Part model, mm, in its own coordinate system. A direction names the side the tool comes from. Round coordinates to 2 decimals unless told otherwise and drop trailing zeros. Order: outer loops, then holes, each group sorted by start corner. A loop starts at its lowest first (then second) coordinate and runs counter-clockwise, first axis right, second up. Notation, with made-up numbers: (64.5, 14) - (111.5, 14) arc R21 ccw to (111.5, 36) - close; hole circle Ø8 at (16.5, 25.25). An arc over 180 degrees is marked (long way). Return JSON: item names as keys, results as strings. Group by question number.
Item 1: Tool access for faces 1 (the face through (-32.795, -70.53, 4.698)), 2 (the face through (30.354, -69.132, 4.698)), 3 (the face through (41.99, -80.98, 0.49)): list every direction of +Z, -Z, +X, -X, +Y, -Y with a clear straight run to the whole face (end or side of a thin tool).
Item 2: Saw through at C-C on z = 2.5. State how many separate pieces and enclosed holes the cut face has, and give its area (3 significant figures).
Item 3: Probe probe 1 along X at (y, z) = (12, 4.25); probe 2 along Z at (x, y) = (38.5, -73.5); probe 3 along X at (y, z) = (3, 1.75). List the from-to ranges inside material, lowest first.
Item 4: Saw through at B-B on y = 26.5. List the corners of the cut face in (x, z), and give its area (3 significant figures).
Item 5: Drop flat-ended pins along their axis: pin 1 (2 mm diameter, centred on y = -13, z = 3, fed in from +X); pin 2 (4 mm diameter, centred on y = -7, z = 3.5, fed in from -X); pin 3 (3 mm diameter, centred on x = 13.5, z = 3.5, fed in from -Y). Give the stop position or say it passes through.
Item 6: Two-plate mould, pull along Y, no slides. Class faces 4 (the face through (-32.506, -44, 5)), 5 (the face through (-43, 49.31, 0.49)), 6 (the face through (-34.506, -15, 5)): released by +Y, released by -Y, zero draft, split by the parting line, or undercut.
```python
from build123d import *

# Parameters (mm, degrees)
F0_W     = 64
F0_H     = 16.5
F1_DEPTH = 1
F2_DEPTH = 8.5
F0_H_2   = 2
F3_DEPTH = 8.5


with BuildPart() as f1:
    # F0 (on Top) → F1 (new body)
    with BuildSketch(Plane.XY):
        with BuildLine():
            Line((34.994369, 52.165454), (-36.005631, 52.165454))
            ThreePointArc((-36.005631, 52.165454), (-43.076699, 49.236522), (-46.005631, 42.165454))
            Line((-46.005631, 42.165454), (-46.005631, -73.834546))
            ThreePointArc((-46.005631, -73.834546), (-43.076699, -80.905614), (-36.005631, -83.834546))
            Line((-36.005631, -83.834546), (34.994369, -83.834546))
            ThreePointArc((34.994369, -83.834546), (42.065437, -80.905614), (44.994369, -73.834546))
            Line((44.994369, -73.834546), (44.994369, 42.165454))
            ThreePointArc((44.994369, 42.165454), (42.065437, 49.236522), (34.994369, 52.165454))
        make_face()
        with BuildLine():
            ThreePointArc((-38.505631, 34.665454), (-35.576699, 41.736522), (-28.505631, 44.665454))
            Line((-28.505631, 44.665454), (27.494369, 44.665454))
            ThreePointArc((27.494369, 44.665454), (34.565437, 41.736522), (37.494369, 34.665454))
            Line((37.494369, 34.665454), (37.494369, -66.334546))
            ThreePointArc((37.494369, -66.334546), (34.565437, -73.405614), (27.494369, -76.334546))
            Line((27.494369, -76.334546), (-28.505631, -76.334546))
            ThreePointArc((-28.505631, -76.334546), (-35.576699, -73.405614), (-38.505631, -66.334546))
            Line((-38.505631, -66.334546), (-38.505631, 34.665454))
        make_face(mode=Mode.SUBTRACT)
        with BuildLine():
            Line((27.494369, 44.665454), (-28.505631, 44.665454))
            ThreePointArc((-28.505631, 44.665454), (-35.576699, 41.736522), (-38.505631, 34.665454))
            Line((-38.505631, 34.665454), (-38.505631, -66.334546))
            ThreePointArc((-38.505631, -66.334546), (-35.576699, -73.405614), (-28.505631, -76.334546))
            Line((-28.505631, -76.334546), (27.494369, -76.334546))
            ThreePointArc((27.494369, -76.334546), (34.565437, -73.405614), (37.494369, -66.334546))
            Line((37.494369, -66.334546), (37.494369, 34.665454))
            ThreePointArc((37.494369, 34.665454), (34.565437, 41.736522), (27.494369, 44.665454))
        make_face()
        with BuildLine():
            ThreePointArc((-36.505631, 34.665454), (-34.162485, 40.322309), (-28.505631, 42.665454))
            Line((-28.505631, 42.665454), (27.494369, 42.665454))
            ThreePointArc((27.494369, 42.665454), (33.151223, 40.322309), (35.494369, 34.665454))
            Line((35.494369, 34.665454), (35.494369, -66.334546))
            ThreePointArc((35.494369, -66.334546), (33.151223, -71.9914), (27.494369, -74.334546))
            Line((27.494369, -74.334546), (-28.505631, -74.334546))
            ThreePointArc((-28.505631, -74.334546), (-34.162485, -71.9914), (-36.505631, -66.334546))
            Line((-36.505631, -66.334546), (-36.505631, 34.665454))
        make_face(mode=Mode.SUBTRACT)
        with BuildLine():
            Line((27.494369, 42.665454), (-28.505631, 42.665454))
            ThreePointArc((-28.505631, 42.665454), (-34.162485, 40.322309), (-36.505631, 34.665454))
            Line((-36.505631, 34.665454), (-36.505631, -66.334546))
            ThreePointArc((-36.505631, -66.334546), (-34.162485, -71.9914), (-28.505631, -74.334546))
            Line((-28.505631, -74.334546), (27.494369, -74.334546))
            ThreePointArc((27.494369, -74.334546), (33.151223, -71.9914), (35.494369, -66.334546))
            Line((35.494369, -66.334546), (35.494369, 34.665454))
            ThreePointArc((35.494369, 34.665454), (33.151223, 40.322309), (27.494369, 42.665454))
        make_face()
        with BuildLine():
            ThreePointArc((-34.505631, 34.665454), (-32.748272, 38.908095), (-28.505631, 40.665454))
            Line((-28.505631, 40.665454), (27.494369, 40.665454))
            ThreePointArc((27.494369, 40.665454), (31.73701, 38.908095), (33.494369, 34.665454))
            Line((33.494369, 34.665454), (33.494369, -66.334546))
            ThreePointArc((33.494369, -66.334546), (31.73701, -70.577186), (27.494369, -72.334546))
            Line((27.494369, -72.334546), (-28.505631, -72.334546))
            ThreePointArc((-28.505631, -72.334546), (-32.748272, -70.577186), (-34.505631, -66.334546))
            Line((-34.505631, -66.334546), (-34.505631, 34.665454))
        make_face(mode=Mode.SUBTRACT)
        with BuildLine():
            Line((27.494369, 40.665454), (-28.505631, 40.665454))
            ThreePointArc((-28.505631, 40.665454), (-32.748272, 38.908095), (-34.505631, 34.665454))
            Line((-34.505631, 34.665454), (-34.505631, -66.334546))
            ThreePointArc((-34.505631, -66.334546), (-32.748272, -70.577186), (-28.505631, -72.334546))
            Line((-28.505631, -72.334546), (27.494369, -72.334546))
            ThreePointArc((27.494369, -72.334546), (31.73701, -70.577186), (33.494369, -66.334546))
            Line((33.494369, -66.334546), (33.494369, 34.665454))
            ThreePointArc((33.494369, 34.665454), (31.73701, 38.908095), (27.494369, 40.665454))
        make_face()
        with BuildLine():
            ThreePointArc((-32.505631, 34.665454), (-31.334058, 37.493881), (-28.505631, 38.665454))
            Line((-28.505631, 38.665454), (27.494369, 38.665454))
            ThreePointArc((27.494369, 38.665454), (30.322796, 37.493881), (31.494369, 34.665454))
            Line((31.494369, 34.665454), (31.494369, 22.165454))
            Line((31.494369, 22.165454), (31.494369, 20.165454))
            Line((31.494369, 20.165454), (31.494369, 3.665454))
            Line((31.494369, 3.665454), (31.494369, 1.665454))
            Line((31.494369, 1.665454), (31.494369, -14.834546))
            Line((31.494369, -14.834546), (31.494369, -16.834546))
            Line((31.494369, -16.834546), (31.494369, -33.334546))
            Line((31.494369, -33.334546), (31.494369, -35.334546))
            Line((31.494369, -35.334546), (31.494369, -51.834546))
            Line((31.494369, -51.834546), (31.494369, -53.834546))
            Line((31.494369, -53.834546), (31.494369, -66.334546))
            ThreePointArc((31.494369, -66.334546), (30.322796, -69.162973), (27.494369, -70.334546))
            Line((27.494369, -70.334546), (-28.505631, -70.334546))
            ThreePointArc((-28.505631, -70.334546), (-31.334058, -69.162973), (-32.505631, -66.334546))
            Line((-32.505631, -66.334546), (-32.505631, -53.834546))
            Line((-32.505631, -53.834546), (-32.505631, -51.834546))
            Line((-32.505631, -51.834546), (-32.505631, -35.334546))
            Line((-32.505631, -35.334546), (-32.505631, -33.334546))
            Line((-32.505631, -33.334546), (-32.505631, -16.834546))
            Line((-32.505631, -16.834546), (-32.505631, -14.834546))
            Line((-32.505631, -14.834546), (-32.505631, 1.665454))
            Line((-32.505631, 1.665454), (-32.505631, 3.665454))
            Line((-32.505631, 3.665454), (-32.505631, 20.165454))
            Line((-32.505631, 20.165454), (-32.505631, 22.165454))
            Line((-32.505631, 22.165454), (-32.505631, 34.665454))
        make_face(mode=Mode.SUBTRACT)
        with BuildLine():
            Line((27.494369, 38.665454), (-28.505631, 38.665454))
            ThreePointArc((-28.505631, 38.665454), (-31.334058, 37.493881), (-32.505631, 34.665454))
            Line((-32.505631, 34.665454), (-32.505631, 22.165454))
            Line((-32.505631, 22.165454), (31.494369, 22.165454))
            Line((31.494369, 22.165454), (31.494369, 34.665454))
            ThreePointArc((31.494369, 34.665454), (30.322796, 37.493881), (27.494369, 38.665454))
        make_face()
        with Locations((-0.505631, 11.915454)):
            Rectangle(F0_W, F0_H)
        with Locations((-0.505631, -6.584546)):
            Rectangle(F0_W, F0_H)
        with Locations((-0.505631, -25.084546)):
            Rectangle(F0_W, F0_H)
        with Locations((-0.505631, -43.584546)):
            Rectangle(F0_W, F0_H)
        with BuildLine():
            Line((31.494369, -53.834546), (-32.505631, -53.834546))
            Line((-32.505631, -53.834546), (-32.505631, -66.334546))
            ThreePointArc((-32.505631, -66.334546), (-31.334058, -69.162973), (-28.505631, -70.334546))
            Line((-28.505631, -70.334546), (27.494369, -70.334546))
            ThreePointArc((27.494369, -70.334546), (30.322796, -69.162973), (31.494369, -66.334546))
            Line((31.494369, -66.334546), (31.494369, -53.834546))
        make_face()
    extrude(amount=F1_DEPTH)



with BuildPart() as f2:
    # F0 (on Top) → F2 (new body)
    with BuildSketch(Plane.XY):
        with BuildLine():
            Line((27.494369, 40.665454), (-28.505631, 40.665454))
            ThreePointArc((-28.505631, 40.665454), (-32.748272, 38.908095), (-34.505631, 34.665454))
            Line((-34.505631, 34.665454), (-34.505631, -66.334546))
            ThreePointArc((-34.505631, -66.334546), (-32.748272, -70.577186), (-28.505631, -72.334546))
            Line((-28.505631, -72.334546), (27.494369, -72.334546))
            ThreePointArc((27.494369, -72.334546), (31.73701, -70.577186), (33.494369, -66.334546))
            Line((33.494369, -66.334546), (33.494369, 34.665454))
            ThreePointArc((33.494369, 34.665454), (31.73701, 38.908095), (27.494369, 40.665454))
        make_face()
        with BuildLine():
            ThreePointArc((-32.505631, 34.665454), (-31.334058, 37.493881), (-28.505631, 38.665454))
            Line((-28.505631, 38.665454), (27.494369, 38.665454))
            ThreePointArc((27.494369, 38.665454), (30.322796, 37.493881), (31.494369, 34.665454))
            Line((31.494369, 34.665454), (31.494369, 22.165454))
            Line((31.494369, 22.165454), (31.494369, 20.165454))
            Line((31.494369, 20.165454), (31.494369, 3.665454))
            Line((31.494369, 3.665454), (31.494369, 1.665454))
            Line((31.494369, 1.665454), (31.494369, -14.834546))
            Line((31.494369, -14.834546), (31.494369, -16.834546))
            Line((31.494369, -16.834546), (31.494369, -33.334546))
            Line((31.494369, -33.334546), (31.494369, -35.334546))
            Line((31.494369, -35.334546), (31.494369, -51.834546))
            Line((31.494369, -51.834546), (31.494369, -53.834546))
            Line((31.494369, -53.834546), (31.494369, -66.334546))
            ThreePointArc((31.494369, -66.334546), (30.322796, -69.162973), (27.494369, -70.334546))
            Line((27.494369, -70.334546), (-28.505631, -70.334546))
            ThreePointArc((-28.505631, -70.334546), (-31.334058, -69.162973), (-32.505631, -66.334546))
            Line((-32.505631, -66.334546), (-32.505631, -53.834546))
            Line((-32.505631, -53.834546), (-32.505631, -51.834546))
            Line((-32.505631, -51.834546), (-32.505631, -35.334546))
            Line((-32.505631, -35.334546), (-32.505631, -33.334546))
            Line((-32.505631, -33.334546), (-32.505631, -16.834546))
            Line((-32.505631, -16.834546), (-32.505631, -14.834546))
            Line((-32.505631, -14.834546), (-32.505631, 1.665454))
            Line((-32.505631, 1.665454), (-32.505631, 3.665454))
            Line((-32.505631, 3.665454), (-32.505631, 20.165454))
            Line((-32.505631, 20.165454), (-32.505631, 22.165454))
            Line((-32.505631, 22.165454), (-32.505631, 34.665454))
        make_face(mode=Mode.SUBTRACT)
    extrude(amount=F2_DEPTH)


with BuildPart() as f1_1:
    add(f1.part)

    add(f2.part)  # F3 merges F2
    # F0 (on Top) → F3 (join)
    with BuildSketch(Plane.XY):
        with Locations((-0.505631, 21.165454)):
            Rectangle(F0_W, F0_H_2)
        with Locations((-0.505631, 2.665454)):
            Rectangle(F0_W, F0_H_2)
        with Locations((-0.505631, -15.834546)):
            Rectangle(F0_W, F0_H_2)
        with Locations((-0.505631, -34.334546)):
            Rectangle(F0_W, F0_H_2)
        with Locations((-0.505631, -52.834546)):
            Rectangle(F0_W, F0_H_2)
    extrude(amount=F3_DEPTH)


solid = f1_1.part
```
Filled in:
{
 "1": {"face 1": "+Z, -X, -Y", "face 2": "+Z", "face 3": "+Z, -Z, +X, -Y"},
 "2": {"separate pieces": "1", "enclosed holes": "6", "area": "1,330 mm^2"},
 "3": {"probe 1": "x = -34.51 to -32.51, 31.49 to 33.49", "probe 2": "z = 0 to 1", "probe 3": "x = -34.51 to 33.49"},
 "4": {"outline": "(-46.01, 0) - (44.99, 0) - (44.99, 1) - (33.49, 1) - (33.49, 8.5) - (31.49, 8.5) - (31.49, 1) - (-32.51, 1) - (-32.51, 8.5) - (-34.51, 8.5) - (-34.51, 1) - (-46.01, 1) - close", "area": "121 mm^2"},
 "5": {"pin 1": "stops at x = 33.49", "pin 2": "stops at x = -34.51", "pin 3": "stops at y = -72.33"},
 "6": {"face 4": "undercut", "face 5": "released by +Y", "face 6": "zero draft"}
}
